Print and shaded views of the part. All mm, measured from the part's lowest x, y and z. Coordinates: 2 decimals unless noted, no trailing zeros. Order: outer loops, then holes, each group sorted by start corner. A loop starts at its lowest first (then second) coordinate and runs counter-clockwise, first axis right, second up. Notation, with made-up numbers: (0, -5.5) -> (34, -5.5) arc R24 ccw to (34, 27.5) -> close; hole circle Ø9 at (81.25, -13). An arc over 180 degrees is marked (long way). Write item = value, one per line. Start each with the question number.
Q1. Cut at C-C, the plane z = 35. List the corners of the cut face in (x, y).
Q2. Cut at A-A, the plane y = 0.8. List the corners of the cut face in (x, z), plus the area to 3 significant figures.
Q3. Wall check: line 1 (X direction, y = 0.4, z = 23); line 2 (Z direction, x = 61, y = 0.45). Give the ranges that are in metal, low to high. Write a range as from..to.
Q4. Cut at B-B, the plane x = 82.5. List the corners of the cut face in (y, z).
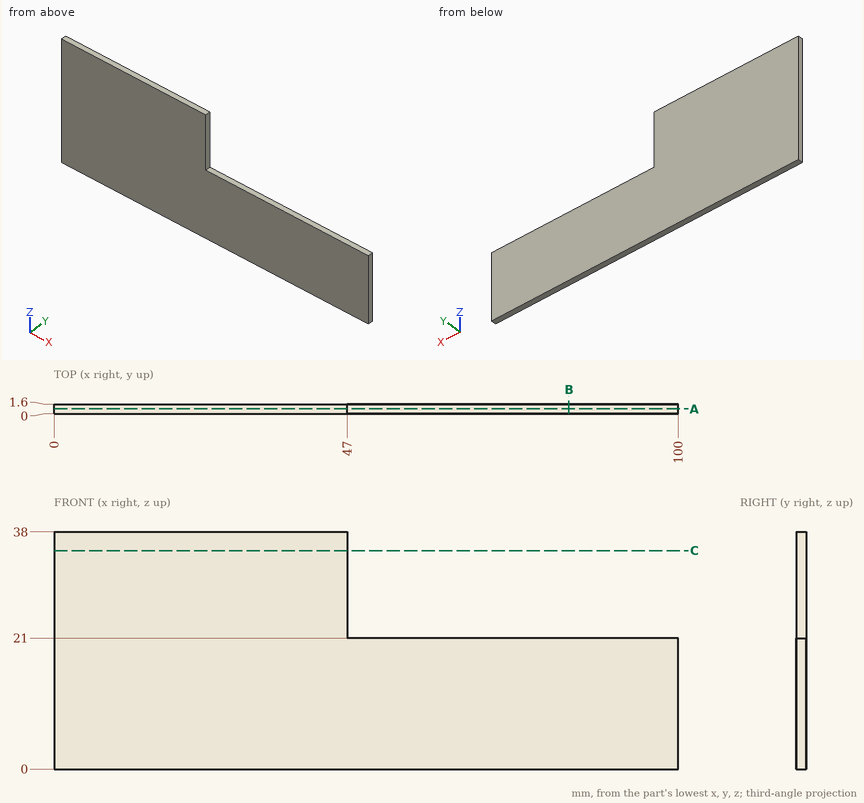
Here are the results:
q1.outline = (0, 0) -> (47, 0) -> (47, 1.6) -> (0, 1.6) -> close
q2.outline = (0, 0) -> (100, 0) -> (100, 21) -> (47, 21) -> (47, 38) -> (0, 38) -> close
q2.area = 2,900 mm²
q3.line_1 = 0..47
q3.line_2 = 0..21
q4.outline = (0, 0) -> (1.6, 0) -> (1.6, 21) -> (0, 21) -> close
